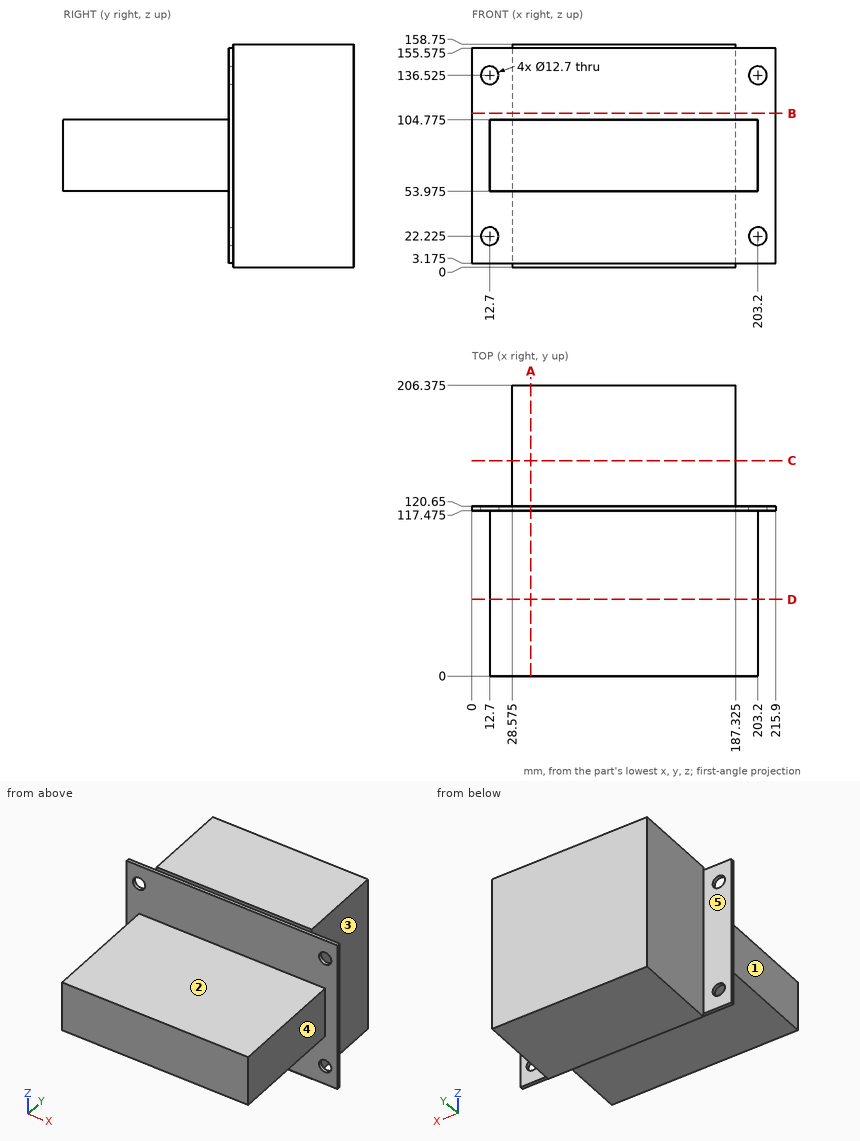
Here's the drawing with two shaded views (mm, measured from the low corner). I have some questions. A direction names the side the tool comes from. Coordinates: 2 decimals unless noted, no trailing zeros. Write each loop counter-clockwise with the first axis right and the second up, starting at its lowest first coordinate (ties: lowest second). Pieces come first, ordered by that corner, then holes. Notation, with made-up numbers: (-13, 29) -> (1, 29) arc R27 cw to (1, 46) -> close; hole circle Ø6 at (-22.5, -9.5). An arc over 180 degrees is marked (long way). Write item = value, one per line. Start each with the question number.
(1) I want a section at C-C (y = 153). Please give me the cut outline in (x, z) (3 decimals), plus the area to 3 significant figures.
(2) I want a section at B-B (z = 109.5). Please give me the cut outline in (x, y) (3 decimals), plus the area to 3 significant figures.
(3) I need wall thicknesses on line 1 (Z direction, x = 12, y = 118) (3 decimals); line 2 (Z direction, x = 12.7, y = 119.8) (3 decimals); line 3 (X direction, y = 183.5, z = 55) (3 decimals). Which ranges of each line are inside material? Lowest first, please. Write a range as [from, to].
(4) I want a section at A-A (x = 42). Please give me the cut outline in (y, z) (3 decimals), plus the area to 3 significant figures.
(5) Will these pins go through, and if not, where does the flat tip stop? pin 1 (12 mm diameter, centred on y = 137, z = 91.5, fed in from -X) (3 decimals); pin 2 (1.5 mm diameter, centred on y = 21.5, z = 102.5, fed in from -X); pin 3 (1 mm diameter, centred on x = 85, z = 157.5, fed in from -Y).
(6) I want a section at D-D (y = 54.5). Please give me the cut outline in (x, z) (3 decimals).
(7) Which directions (+Z, -Z, +X, -X, +Y, -Y) give clear straight access to the entire face, cutting with the end or side of a thin tool? Please do the marked faces 1, 2, 3, 4 and 5.
Result set:
q1.outline = (28.575, 0) -> (187.325, 0) -> (187.325, 158.75) -> (28.575, 158.75) -> close
q1.area = 25,200 mm2
q2.outline = (0, 117.475) -> (215.9, 117.475) -> (215.9, 120.65) -> (187.325, 120.65) -> (187.325, 206.375) -> (28.575, 206.375) -> (28.575, 120.65) -> (0, 120.65) -> close
q2.area = 14,300 mm2
q3.line_1 = [3.175, 15.914], [28.536, 130.214], [142.836, 155.575]
q3.line_2 = [3.175, 15.875], [28.575, 130.175], [142.875, 155.575]
q3.line_3 = [28.575, 187.325]
q4.outline = (0, 53.975) -> (117.475, 53.975) -> (117.475, 3.175) -> (120.65, 3.175) -> (120.65, 0) -> (206.375, 0) -> (206.375, 158.75) -> (120.65, 158.75) -> (120.65, 155.575) -> (117.475, 155.575) -> (117.475, 104.775) -> (0, 104.775) -> close
q4.area = 20,100 mm2
q5.pin_1 = 28.575
q5.pin_2 = 12.7
q5.pin_3 = 120.65
q6.outline = (12.7, 53.975) -> (203.2, 53.975) -> (203.2, 104.775) -> (12.7, 104.775) -> close
q7.face_1 = +Z, -Z, -X, -Y
q7.face_2 = +Z, +X, -X, -Y
q7.face_3 = +Z, -Z, +X, +Y
q7.face_4 = +Z, -Z, +X, -Y
q7.face_5 = +Z, -Z, -X, +Y
